Could you check a few things on this model? Use its own coordinates, in mm. Face numbers are marked on the shaded views. Give positions to 0.01 mm unless a question says otherwise; leave off trailing zeros. Write each loop counter-clockwise with the first axis right and the second up, starting at its lowest first coordinate (ties: lowest second). Pieces come first, ordered by that corner, then holes. Notation, with made-up numbers: (42.25, -25.5) - (61.25, -25.5) arc R30 cw to (61.25, 2.5) - close; hole circle Ø7 at (78, 57.25). An arc over 180 degrees is marked (long way). Answer as CSV lines item,"result". Start each with the question number.
Q1. Imagine slicing it at C-C on z = 1. State how many separate pieces and enclosed holes the cut face has, and give its area (3 significant figures).
Q2. Imagine slicing it at B-B on x = 16. List the corners of the cut face in (y, z) for me, and give its area (3 significant figures).
Q3. We'd pull the mould along X, two halves only. Please class the marked faces 1, 2 and 3: pulls with the +X half, pulls with the -X half, needs draft (parallel to the pull), parting line crosses it, or undercut.
Q4. Will these pins go through, and if not, where does the flat tip stop? pin 1 Ø2.5 at (x, y) = (8, -8) entering from -Z; pin 2 Ø8 at (x, z) = (16, 2.5) entering from -Y; pin 3 Ø1 at (x, z) = (-18, 3) entering from +Y; pin 4 Ø3 at (x, y) = (-22.5, 6) entering from +Z.
Q5. Imagine slicing it at A-A on z = 10.25. List the corners of the cut face in (x, y) for me.
Q6. If I drill on line 1 along Y through (x, z) = (-16, -2.5); line 2 along X through (y, z) = (-14.5, 1.5); line 3 along Y through (x, z) = (8, 0.25), over which ranges is the centre line in solid material (lowest first)?
Q7. Imagine slicing it at D-D on y = 24. List the corners of the cut face in (x, z) for me, and give its area (3 significant figures).
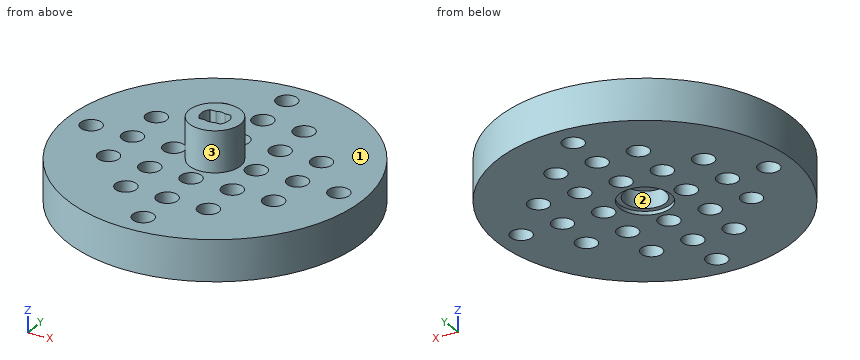
```python
from build123d import *

# Parameters (mm, degrees)
SKETCH_1_R               = 28.85
EXTRUDE_1_DEPTH          = 4
EXTRUDE_1_DEPTH_BACK     = 4
SKETCH_2_R               = 5
EXTRUDE_2_DEPTH          = 8
SKETCH_3_R               = 1.8
CUT_EXTRUDE_1_DEPTH      = 44.825164004
SKETCH_4_R               = 4
CUT_EXTRUDE_2_DEPTH      = 4
SKETCH_5_R               = 5
CUT_EXTRUDE_3_DEPTH      = 0.7
CUT_EXTRUDE_4_DEPTH      = 7.5
SKETCH_7_R               = 2.05
CUT_EXTRUDE_5_DEPTH      = 43.528167137
CUT_EXTRUDE_5_DEPTH_BACK = 43.528167137


with BuildPart() as part:
    # Sketch 1 → Extrude 1 (new, two sides)
    with BuildSketch(Plane.XY) as extrude_1_sk:
        Circle(SKETCH_1_R)
    extrude(amount=EXTRUDE_1_DEPTH)
    extrude(extrude_1_sk.sketch, amount=-EXTRUDE_1_DEPTH_BACK)

    # Sketch 2 → Extrude 2 (add)
    with BuildSketch(Plane.XY.offset(4)):
        Circle(SKETCH_2_R)
    extrude(amount=EXTRUDE_2_DEPTH)

    # Sketch 3 → Cut-Extrude 1 (cut, through all)
    with BuildSketch(Plane.XY.offset(12)):
        Circle(SKETCH_3_R)
    extrude(amount=-CUT_EXTRUDE_1_DEPTH, mode=Mode.SUBTRACT)

    # Sketch 4 → Cut-Extrude 2 (cut)
    with BuildSketch(Plane(origin=(0, 0, -4), x_dir=(-1, 0, 0), z_dir=(0, 0, -1))):
        Circle(SKETCH_4_R)
    extrude(amount=-CUT_EXTRUDE_2_DEPTH, mode=Mode.SUBTRACT)

    # Sketch 5 → Cut-Extrude 3 (cut)
    with BuildSketch(Plane(origin=(0, 0, -4), x_dir=(-1, 0, 0), z_dir=(0, 0, -1))):
        with Locations(Location((0, 0, 0), (0, 0, 180))):
            Circle(SKETCH_5_R)
    extrude(amount=-CUT_EXTRUDE_3_DEPTH, mode=Mode.SUBTRACT)

    # Sketch 6 → Cut-Extrude 4 (cut)
    with BuildSketch(Plane.XY.offset(12)):
        with BuildLine():
            ThreePointArc((2.01246118, -1.8), (2.7, 0), (2.01246118, 1.8))
            Line((2.01246118, 1.8), (0.871779789, 1.8))
            ThreePointArc((0.871779789, 1.8), (0, 2), (-0.871779789, 1.8))
            Line((-0.871779789, 1.8), (-2.01246118, 1.8))
            ThreePointArc((-2.01246118, 1.8), (-2.7, 0), (-2.01246118, -1.8))
            Line((-2.01246118, -1.8), (-0.871779789, -1.8))
            ThreePointArc((-0.871779789, -1.8), (0, -2), (0.871779789, -1.8))
            Line((0.871779789, -1.8), (2.01246118, -1.8))
        make_face()
    extrude(amount=-CUT_EXTRUDE_4_DEPTH, mode=Mode.SUBTRACT)

    # Sketch 7 → Cut-Extrude 5 (cut, two sides)
    with BuildSketch(Plane.XY) as cut_extrude_5_sk:
        with Locations((-24, 0)):
            Circle(SKETCH_7_R)
        with Locations((-16, 0)):
            Circle(SKETCH_7_R)
        with Locations((-8, 0)):
            Circle(SKETCH_7_R)
        with Locations((-8, 8)):
            Circle(SKETCH_7_R)
        with Locations((-16, 8)):
            Circle(SKETCH_7_R)
        with Locations((0, 8)):
            Circle(SKETCH_7_R)
        with Locations((0, 16)):
            Circle(SKETCH_7_R)
        with Locations((-8, 16)):
            Circle(SKETCH_7_R)
        with Locations((0, 24)):
            Circle(SKETCH_7_R)
        with Locations((0, -24)):
            Circle(SKETCH_7_R)
        with Locations((-8, -16)):
            Circle(SKETCH_7_R)
        with Locations((0, -16)):
            Circle(SKETCH_7_R)
        with Locations((0, -8)):
            Circle(SKETCH_7_R)
        with Locations((-16, -8)):
            Circle(SKETCH_7_R)
        with Locations((-8, -8)):
            Circle(SKETCH_7_R)
        with Locations((8, -8)):
            Circle(SKETCH_7_R)
        with Locations((16, -8)):
            Circle(SKETCH_7_R)
        with Locations((8, -16)):
            Circle(SKETCH_7_R)
        with Locations((8, 16)):
            Circle(SKETCH_7_R)
        with Locations((16, 8)):
            Circle(SKETCH_7_R)
        with Locations((8, 8)):
            Circle(SKETCH_7_R)
        with Locations((8, 0)):
            Circle(SKETCH_7_R)
        with Locations((16, 0)):
            Circle(SKETCH_7_R)
        with Locations((24, 0)):
            Circle(SKETCH_7_R)
    extrude(amount=CUT_EXTRUDE_5_DEPTH, mode=Mode.SUBTRACT)
    extrude(cut_extrude_5_sk.sketch, amount=-CUT_EXTRUDE_5_DEPTH_BACK, mode=Mode.SUBTRACT)


solid = part.part
```
Conclusion:
1,separate pieces,"1"
1,enclosed holes,"25"
1,area,"2,290 mm^2"
2,outline,"(-24.01, -4) - (-10.05, -4) - (-10.05, 4) - (-24.01, 4) - close; (-5.95, -4) - (-2.05, -4) - (-2.05, 4) - (-5.95, 4) - close; (2.05, -4) - (5.95, -4) - (5.95, 4) - (2.05, 4) - close; (10.05, -4) - (24.01, -4) - (24.01, 4) - (10.05, 4) - close"
2,area,"286 mm^2"
3,face 1,"needs draft"
3,face 2,"undercut"
3,face 3,"parting line crosses it"
4,pin 1,"through"
4,pin 2,"y = -26.24"
4,pin 3,"y = 22.94"
4,pin 4,"z = 4"
5,outline,"circle Ø10 at (0, 0); hole (-2.01, -1.8) - (-0.87, -1.8) arc R2 ccw to (0.87, -1.8) - (2.01, -1.8) arc R2.7 ccw to (2.01, 1.8) - (0.87, 1.8) arc R2 ccw to (-0.87, 1.8) - (-2.01, 1.8) arc R2.7 ccw to start"
6,line 1,"-24.01 to -10.05, -5.95 to -2.05, 2.05 to 5.95, 10.05 to 24.01"
6,line 2,"-24.94 to -9.4, -6.6 to -1.4, 1.4 to 6.6, 9.4 to 24.94"
6,line 3,"-27.72 to -18.05, -13.95 to -10.05, -5.95 to -2.05, 2.05 to 5.95, 10.05 to 13.95, 18.05 to 27.72"
7,outline,"(-16.01, -4) - (-2.05, -4) - (-2.05, 4) - (-16.01, 4) - close; (2.05, -4) - (16.01, -4) - (16.01, 4) - (2.05, 4) - close"
7,area,"223 mm^2"
